Design review of the part built by this model. Coordinates are the model's own, in mm. A direction names the side the tool comes from. Give positions to 0.01 mm unless a question says otherwise; leave off trailing zeros. Loops run counter-clockwise (first coordinate to the right, second up) from the corner with the lowest first, then second, coordinate; pieces in that order, holes last. Notation, with made-up numbers: M 34.25,-35.5 L 85.25,-35.5 A7 ccw 85.25,-24.5 Z; hole C -38,24.5 d6. An arc over 180 degrees is marked long. Use CSV: the item, a comma, the result in double quotes.
from build123d import *

# Parameters (mm, degrees)
REVOLVE1_ANGLE = 180


with BuildPart() as part:
    # Sketch1 → Revolve1 (revolve)
    with BuildSketch(Plane.XY):
        with BuildLine():
            Line((-3.3655, 1.5875), (-3.3655, 3.175))
            Line((-3.3655, 3.175), (-5.93725, 3.175))
            Line((-5.93725, 3.175), (-4.746625, -2.38125))
            Line((-4.746625, -2.38125), (-3.3655, -2.38125))
            Line((-3.3655, -2.38125), (-3.3655, -1.5875))
            Line((-3.3655, -1.5875), (-2.407358992, -0.629358992))
            ThreePointArc((-2.407358992, -0.629358992), (-2.235295621, -0.371847959), (-2.174875, -0.068092985))
            Line((-2.174875, -0.068092985), (-2.174875, 0.79375))
            ThreePointArc((-2.174875, 0.79375), (-2.407358992, 1.355016008), (-2.968625, 1.5875))
            Line((-2.968625, 1.5875), (-3.3655, 1.5875))
        make_face()
    revolve(axis=Axis((0, 1.5875, 0), (0, -1, 0)), revolution_arc=REVOLVE1_ANGLE)


solid = part.part
(1) We need section C-C on y = 2.8. State the section outline as (x, z) points, then the cut area to 3 significant figures.
A:
outline,"M -5.86,0 A5.86 ccw 5.86,0 L 3.37,0 A3.37 cw -3.37,0 Z"
area,"36.1 mm²"
(2) We need section B-B on y = -1.8. State the section outline as (x, z) points.
A:
outline,"M -4.87,0 A4.87 ccw 4.87,0 L 3.37,0 A3.37 cw -3.37,0 Z"
(3) The part is to be moulded in two halves that separate along X. For faces 1 (the conical face through (-0.11, -0.26, -5.2)), 2 (the flat face through (-4, 0, 0)), 3 (the flat face through (-1, 1.588, -3)), say which applies: released by +X, released by -X, zero draft, split by the parting line, or undercut.
A:
face 1,"split by the parting line"
face 2,"zero draft"
face 3,"undercut"
(4) Wall thickness on line 1 along X through (y, z) = (2.35, -2.9); line 2 along X through (y, z) = (-1.4, -2.2); line 3 along Z through (x, y) = (-2.25, -2.05): over which ranges is each line inside the solid? List them lowest first. Write a range as [from, to].
A:
line 1,"[-4.98, -1.71], [1.71, 4.98]"
line 2,"[-4.44, -2.29], [2.29, 4.44]"
line 3,"[-4.26, -2.5]"
(5) Clearance check with flat-ended pins moving along their axes: P1, Ø1.5, axis at x = -0.5, z = -1.5, coming from the -Y side; P2, Ø2.5, axis at x = 1.5, z = -2, coming from the +Y side (3 decimals); P3, Ø1, axis at y = 2.5, z = -1.5, coming from the -X side. State where each tip first meets the part, or that it passes through.
A:
P1,"y = -0.54"
P2,"y = 3.175"
P3,"x = -5.76"
(6) Machinability: for faces 4 (the cylindrical face through (-0.074, -1.979, -3.365)), 5 (the cylindrical face through (-0.048, 0.369, -2.174)), 6 (the cylindrical face through (-0.074, 2.392, -3.365)), which of the approach directions +Z, -Z, +X, -X, +Y, -Y give a long, thin tool a straight path to every point of the face, cutting with its end or side? Answer none if there is none.
A:
face 4,"+Z, -Y"
face 5,"+Z, +Y, -Y"
face 6,"+Z, +Y"
